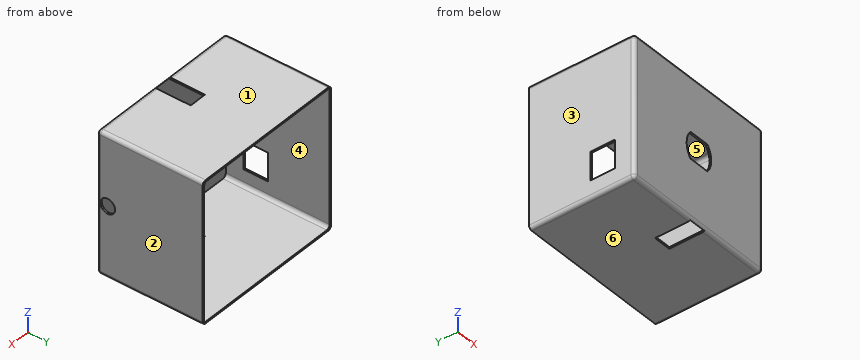
Autodesk Inventor part; units mm, degrees
ref_plane "YZ Plane" through (0, 0, 0) normal (1, 0, 0) x (0, 1, 0)
ref_plane "XZ Plane" through (0, 0, 0) normal (0, 1, 0) x (-1, 0, 0)
ref_plane "XY Plane" through (0, 0, 0) normal (0, 0, 1) x (1, 0, 0)
sketch "Esquisse1" plane through (0, 0, 0) normal (1, 0, 0) x (0, 1, 0)
  line L0 (0, 0) -> (60, 0)
  line L1 (60, 0) -> (60, -80)
  line L2 (60, -80) -> (0, -80)
  line L3 (0, -80) -> (0, 0)
  line L4 (0, -45) -> (0, -35)
  line L5 (0, -35) -> (0, -45)
  point P0 (12.5, -45)
  point P1 (0, -40)
  point P2 (0, -40)
  dimension "d0" = 80
  dimension "d1" = 60
  dimension "d4" = 40
extrude "Extrusion1" add sketch "Esquisse1" along normal blind 90
sketch "Esquisse2" plane through (0, 0, 0) normal (-1, 0, 0) x (0, 0, 1)
  line L0 (0, 0) -> (-80, 0)
  line L1 (-45, 0) -> (-35, 0)
  line L2 (0, 0) -> (-80, 0)
  point P0 (-40, 0)
  point P1 (-40, 0)
  point P2 (-40, 1)
  point P3 (-41.0501, 0)
  point P4 (-35, 9.6008)
  point P5 (-45, 11)
  dimension "d9" = 40
  dimension "d14" = 80
shell "Coque1" thickness 1 removed faces 1 at (30, 60, -53.3333)
sketch "Esquisse3" plane through (0, 0, 0) normal (-1, 0, 0) x (0, 0, 1)
  point P0 (0, 0)
sketch "Esquisse4" plane through (0, 0, 0) normal (-1, 0, 0) x (0, 0, 1)
  point P0 (0, 0)
sketch "Esquisse5" plane through (0, 0, -80) normal (0, 0, -1) x (-1, 0, 0)
  line L0 (-50.2889, 1) -> (-40.2889, 1)
  line L1 (-40.2889, 1) -> (-40.2889, 21)
  line L2 (-40.2889, 21) -> (-50.2889, 21)
  line L3 (-50.2889, 21) -> (-50.2889, 1)
  line L4 (0, 0) -> (-90, 0)
  line L5 (0, 0) -> (-90, 0)
  line L6 (-1, 1) -> (-89, 1)
  point P0 (-45, 0)
  point P1 (-40.2889, 0)
  point P2 (-49.4557, 1)
  point P3 (-46.3284, -7.001)
  point P4 (-44.591, 0)
  point P5 (-46.3284, -7.537)
  point P6 (-50.2889, 11)
  point P7 (-50.2889, 11)
  point P8 (-49.5179, 0)
  point P9 (-49.2163, 0)
  dimension "d15" = 10
  dimension "d16" = 20
  dimension "d17" = 1
  dimension "d18" = 88
  dimension "d19" = 90
sketch "Esquisse8" plane through (0, 0, 0) normal (0, 0, 1) x (1, 0, 0)
  point P0 (0, 0)
extrude "Extrusion2" cut sketch "Esquisse5" against normal blind 90
sketch "Esquisse9" plane through (0, 0, 0) normal (-1, 0, 0) x (0, 0, 1)
  line L0 (-50.5224, 1) -> (-50.5224, 2)
  line L1 (-66.5224, 2) -> (-66.5224, 1)
  line L2 (-70.063, 25) -> (-54.063, 25)
  line L3 (-54.063, 25) -> (-54.063, 11)
  line L4 (-54.063, 11) -> (-70.063, 11)
  line L5 (-70.063, 11) -> (-70.063, 25)
  line L6 (0, 0) -> (-80, 0)
  dimension "d23" = 1
  dimension "d24" = 11
  dimension "d25" = 14
  dimension "d26" = 16
extrude "Extrusion3" cut sketch "Esquisse9" against normal blind 50
sketch "Esquisse10" plane through (90, 0, 0) normal (1, 0, 0) x (0, 0, -1)
  circle A0 centre (39.7201, 6) radius 4.1979
  line L0 (0, 0) -> (80, 0)
  dimension "d29" = 6
extrude "Extrusion4" cut sketch "Esquisse10" against normal blind 50
sketch "Esquisse11" plane through (0, 0, -80) normal (0, -1, 0) x (1, 0, 0)
  line L0 (39.1611, 33.4845) -> (51.1611, 33.4845)
  line L1 (51.1611, 33.4845) -> (51.1611, 48.4845)
  line L2 (51.1611, 48.4845) -> (39.1611, 48.4845)
  line L3 (39.1611, 48.4845) -> (39.1611, 33.4845)
  arc A0 (39.1611, 48.4845) -> (39.1611, 33.4845) centre (48.6459, 40.9845) ccw
  arc A1 (51.1611, 33.4845) -> (51.1611, 48.4845) centre (41.7255, 40.9845) ccw
  point P0 (0, 80)
  point P1 (36.5541, 40.9845)
  point P2 (53.7787, 40.9845)
  point P3 (45.1019, 41.2499)
  point P4 (27.4865, 33.4896)
  point P5 (27.0422, 33.4896)
  dimension "d32" = 15
  dimension "d33" = 12
  dimension "d34" = 6.9205
  dimension "d35" = 12.0918
extrude "Extrusion5" cut sketch "Esquisse11" against normal blind 10
fillet "Congé1" radius 2 2 edges at (1, 30.5, -79) (45, 0, -80)
fillet "Congé2" radius 2 2 edges at (90, 30, 0) (45, 0, 0)
fillet "Congé3" radius 2 5 edges at (90, 0.5858, -79.4142) (90, 31, -80) (89.4142, 0.5858, -0.5858) (90, 0, -40) (89, 30.5, -1)
fillet "Congé4" radius 2 5 edges at (0, 0.5858, -79.4142) (0, 31, -80) (0, 0.5858, -0.5858) (0, 31, 0) (0, 0, -40)
properties part number "corps" material "Plastique ABS"
Geometry check sheet. Reference: the model listing, model coordinates, mm. Face numbers are marked on the shaded views. A direction names the side the tool comes from. Round coordinates to 2 decimals unless told otherwise and drop trailing zeros. Order: outer loops, then holes, each group sorted by start corner. A loop starts at its lowest first (then second) coordinate and runs counter-clockwise, first axis right, second up. Notation, with made-up numbers: M 20.25,88.5 L 24.25,88.5 A24 ccw 24.25,124.5 Z; hole C 6,61 d6. An arc over 180 degrees is marked long. Answer as CSV lines item,"result".
1) Gauge pin test, flat ends, axial feed: pin 1 Ø0.8 at (x, z) = (46, -79.5) entering from -Y; pin 2 Ø1.1 at (y, z) = (15.5, -79.5) entering from +X; pin 3 Ø1.1 at (x, y) = (44.5, 0.5) entering from -Z. Record the tip position at first contact, or that the pin passes through.
Entries:
pin 1,"y = 0.33"
pin 2,"x = 89.76"
pin 3,"z = -79.73"
2) Tool access check on the marked faces 5 and 6. Record the directions out of +Z, -Z, +X, -X, +Y, -Y that give a thin tool (end or side, any length) a straight path to the whole face; none if there is none.
Entries:
face 5,"+Y"
face 6,"-Z, +X, -X, +Y, -Y"
3) Mould release check, pull along X, two halves, no side actions. Record for the marked faces 1, 2, 3 and 4: +X half, -X half, draft (parallel to the pull), parting line (faces both ways), or undercut.
Entries:
face 1,"draft"
face 2,"+X half"
face 3,"-X half"
face 4,"undercut"
4) Sectioned sample at A-A on z = -61. Record the cut outline in (x, y), and give its area (3 significant figures).
Entries:
outline,"M 0,2 A2 ccw 2,0 L 88,0 A2 ccw 90,2 L 90,60 L 89,60 L 89,1 L 1,1 L 1,11 L 0,11 Z; M 0,25 L 1,25 L 1,60 L 0,60 Z"
area,"192 mm2"
5) Sectioned sample at D-D on x = 49. Record the cut outline in (y, z).
Entries:
outline,"M 0,-78 A2 ccw 1,-79.73 L 1,-46.52 L 0,-46.52 Z; M 0,-31.52 L 1,-31.52 L 1,-0.27 A2 ccw 0,-2 Z; M 21,-80 L 60,-80 L 60,-79 L 21,-79 Z; M 21,-1 L 60,-1 L 60,0 L 21,0 Z"
6) Thickness scan on probe 1 along Z at (x, y) = (38, 22); probe 2 along X at (y, z) = (54, -45); probe 3 along Y at (x, z) = (79, -61). Record the ranges inside material, lowest first. Write a range as [from, to].
Entries:
probe 1,"[-80, -79], [-1, 0]"
probe 2,"[0, 1], [89, 90]"
probe 3,"[0, 1]"
7) Sectioned sample at B-B on y = 6. Record the cut outline in (x, z).
Entries:
outline,"M 0,-78 A2 ccw 2,-80 L 40.29,-80 L 40.29,-79 L 3,-79 A2 cw 1,-77 L 1,-1 L 40.29,-1 L 40.29,0 L 2,0 A2 ccw 0,-2 Z; M 50.29,-80 L 88,-80 A2 ccw 90,-78 L 90,-43.92 L 89,-43.92 L 89,-79 L 50.29,-79 Z; M 50.29,-1 L 87,-1 A2 cw 89,-3 L 89,-35.52 L 90,-35.52 L 90,-2 A2 ccw 88,0 L 50.29,0 Z"
8) Sectioned sample at C-C on y = 34. Record the cut outline in (x, z).
Entries:
outline,"M 0,-78 A2 ccw 2,-80 L 88,-80 A2 ccw 90,-78 L 90,-2 A2 ccw 88,0 L 2,0 A2 ccw 0,-2 Z; hole M 1,-77 A2 ccw 3,-79 L 89,-79 L 89,-3 A2 ccw 87,-1 L 1,-1 Z"
